from build123d import *

# Parameters (mm, degrees)
SKETCH1_R           = 3
SKETCH1_R_2         = 1.25
SKETCH1_W           = 12
SKETCH1_H           = 4.5
BOSS_EXTRUDE1_DEPTH = 5
CUT_EXTRUDE1_DEPTH  = 2
CUT_EXTRUDE2_DEPTH  = 2.5
CHAMFER1_SIZE       = 1


with BuildPart() as part:
    # Sketch1 → Boss-Extrude1 (new body)
    with BuildSketch(Plane.XY):
        with BuildLine():
            Line((33.192050804, 21), (0, 21))
            Line((0, 21), (0, -72))
            Line((0, -72), (6, -72))
            Line((6, -72), (56.988314669, -60.202043939))
            ThreePointArc((56.988314669, -60.202043939), (80.160384186, -37.165976959), (69.826332353, -6.169000327))
            Line((69.826332353, -6.169000327), (40.227200994, 18.456161174))
            ThreePointArc((40.227200994, 18.456161174), (36.932520499, 20.344509967), (33.192050804, 21))
        make_face()
        with Locations((50, -30)):
            Circle(SKETCH1_R, mode=Mode.SUBTRACT)
        with Locations((70, -30)):
            Circle(SKETCH1_R_2, mode=Mode.SUBTRACT)
        with Locations((15, 9.75)):
            Rectangle(SKETCH1_W, SKETCH1_H, mode=Mode.SUBTRACT)
        with Locations((33.192050804, 10)):
            Circle(SKETCH1_R_2, mode=Mode.SUBTRACT)
        with Locations((10, -59.255419511)):
            Circle(SKETCH1_R_2, mode=Mode.SUBTRACT)
        with Locations((50, -50)):
            Circle(SKETCH1_R_2, mode=Mode.SUBTRACT)
    extrude(amount=BOSS_EXTRUDE1_DEPTH)

    # Sketch2 → Cut-Extrude1 (cut)
    with BuildSketch(Plane.XY.offset(5)):
        Polygon((9, 7.5), (40.725052348, -24.831204578), (46.094372356, -20.126440724), (21, 12), align=None)
    extrude(amount=-CUT_EXTRUDE1_DEPTH, mode=Mode.SUBTRACT)

    # Sketch3 → Cut-Extrude2 (cut)
    with BuildSketch(Plane(origin=(0, 0, 0), x_dir=(-1, 0, 0), z_dir=(0, 0, -1))):
        Polygon((-42.609916554, -30), (-46.304958277, -23.6), (-53.695041723, -23.6), (-57.390083446, -30), (-53.695041723, -36.4), (-46.304958277, -36.4), align=None)
    extrude(amount=-CUT_EXTRUDE2_DEPTH, mode=Mode.SUBTRACT)

    # Chamfer1
    chamfer1_edges = [part.edges().sort_by_distance(p)[0] for p in [
        (21, 9.75, 3),
        (15, 7.5, 3),
    ]]
    chamfer(chamfer1_edges, length=CHAMFER1_SIZE)


solid = part.part
Geometry: final body of the model. Coordinates: model frame, mm. A direction names the side the tool comes from. Give positions to 0.01 mm unless a question says otherwise; leave off trailing zeros. Loops run counter-clockwise (first coordinate to the right, second up) from the corner with the lowest first, then second, coordinate; pieces in that order, holes last. Notation, with made-up numbers: (-10.75, 26) - (48.25, 26) arc R27 ccw to (48.25, 60) - close; hole circle Ø8 at (-28, 51.25). An arc over 180 degrees is marked (long way). Answer as CSV lines item,"result". Start each with the question number.
1. Draft query along Y for faces 1 (the face through (33.723, -4.288, 3.854)), 2 (the face through (36.983, 20.326, 2.465)), 3 (the face through (40, -25, 5)). Return one class per face: released by +Y, released by -Y, zero draft, split by the parting line, or undercut.
2. Reachability of faces 4 (the face through (15, 12, 2)), 5 (the face through (55.52, -26.76, 1.23)), 6 (the face through (17, 21, 2)) from +Z, -Z, +X, -X, +Y, -Y: full face, straight path, thin tool, end or side. Return the list, or none.
3. Section B-B, the plane z = 0.85. Return loops of the section in (x, y).
4. Ray query, L1, parallel to Y at x = 50, z = 4.45; L2, parallel to Y at x = 51.5, z = 2.8; L3, parallel to X at y = -7.5, z = 4.05. Return the intervals inside material, ascending.
5. Section C-C, the plane x = 55.5. Return loops of the section in (y, z).
6. Section A-A, the plane x = 17. Return loops of the section in (y, z), plus the area to 3 significant figures.
7. Section D-D, the plane y = -53. Return loops of the section in (x, z).
8. Pin query (flat end, axial travel): P1, Ø3, axis at y = -28.5, z = 3, coming from the +X side; P2, Ø1.2, axis at x = 50, z = 1.5, coming from the -Y side; P3, Ø1, axis at x = 52, z = 1.5, coming from the -Y side. Return the tip coordinate at first contact, or that it passes through.
Answers:
1,face 1,"undercut"
1,face 2,"released by +Y"
1,face 3,"zero draft"
2,face 4,"+Z, -Z"
2,face 5,"-Z"
2,face 6,"+Z, -Z, +X, -X, +Y"
3,outline,"(0, -72) - (6, -72) - (56.99, -60.2) arc R31 ccw to (69.83, -6.17) - (40.23, 18.46) arc R11 ccw to (33.19, 21) - (0, 21) - close; hole circle Ø2.5 at (10, -59.26); hole (9, 7.5) - (21, 7.5) - (21, 12) - (9, 12) - close; hole circle Ø2.5 at (33.19, 10); hole (42.61, -30) - (46.3, -36.4) - (53.7, -36.4) - (57.39, -30) - (53.7, -23.6) - (46.3, -23.6) - close; hole circle Ø2.5 at (50, -50); hole circle Ø2.5 at (70, -30)"
4,L1,"y = -61.82 to -51.25, -48.75 to -33, -27 to 10.33"
4,L2,"y = -61.47 to -32.6, -27.4 to 9.08"
4,L3,"x = 0 to 23.72, 36.23 to 71.32"
5,outline,"(-60.55, 0) - (-33.27, 0) - (-33.27, 2.5) - (-26.73, 2.5) - (-26.73, 0) - (5.75, 0) - (5.75, 5) - (-60.55, 5) - close"
6,outline,"(-69.45, 0) - (7.5, 0) - (7.5, 2) - (6.5, 3) - (-0.65, 3) - (-0.65, 5) - (-69.45, 5) - close; (12, 0) - (21, 0) - (21, 5) - (12, 5) - close"
6,area,"413 mm2"
7,outline,"(0, 0) - (70.78, 0) - (70.78, 5) - (0, 5) - close"
8,P1,"stops at x = 81"
8,P2,"stops at y = -61.96"
8,P3,"stops at y = -61.47"
